Autodesk Inventor part; units mm, degrees
ref_plane "YZ Plane" through (0, 0, 0) normal (1, 0, 0) x (0, 1, 0)
ref_plane "XZ Plane" through (0, 0, 0) normal (0, 1, 0) x (-1, 0, 0)
ref_plane "XY Plane" through (0, 0, 0) normal (0, 0, 1) x (1, 0, 0)
sketch "Sketch1" plane through (0, 0, 0) normal (0, 1, 0) x (-1, 0, 0)
  line L0 (0, 0) -> (45, 0)
  line L1 (45, 0) -> (45, -20)
  line L2 (45, -20) -> (0, -20)
  line L3 (0, -20) -> (0, 0)
  circle A0 centre (39.9418, -5.8805) radius 1.5
  circle A1 centre (39.4697, -15.8219) radius 1.5
  circle A2 centre (3.2694, -6.6358) radius 1.5
  circle A3 centre (3.2694, -15.8219) radius 1.5
  dimension "d0" = 45
  dimension "d1" = 20
  dimension "d4" = 3
  dimension "d5" = 3
  dimension "d6" = 3
  dimension "d7" = 3
extrude "Extrusion1" add sketch "Sketch1" along normal blind 3 contours L0 L1 L2 L3 | A0 | A1 | A2 | A3
extrude "Extrusion2" cut sketch "Sketch1" along normal through all contours A0 | A1 | A2 | A3
sketch "Sketch2" plane through (-45, 0, 0) normal (0, 0, 1) x (1, 0, 0)
  line L0 (0, 0) -> (45, 0)
  line L1 (45, 0) -> (45, 105)
  line L2 (45, 105) -> (0, 105)
  line L3 (0, 105) -> (0, 0)
  line L4 (10.782, 97.156) -> (34.218, 97.156)
  line L5 (34.218, 97.156) -> (34.218, 84.256)
  line L6 (34.218, 84.256) -> (10.782, 84.256)
  line L7 (10.782, 84.256) -> (10.782, 97.156)
  circle A0 centre (8.582, 90.706) radius 1.5
  circle A1 centre (36.418, 90.706) radius 1.5
  line L8 (10.782, 79.3472) -> (34.218, 79.3472)
  line L9 (34.218, 79.3472) -> (34.218, 66.4472)
  line L10 (34.218, 66.4472) -> (10.782, 66.4472)
  line L11 (10.782, 66.4472) -> (10.782, 79.3472)
  circle A2 centre (8.582, 72.8972) radius 1.5
  circle A3 centre (36.418, 72.8972) radius 1.5
  line L12 (10.782, 61.5315) -> (34.218, 61.5315)
  line L13 (34.218, 61.5315) -> (34.218, 48.6315)
  line L14 (34.218, 48.6315) -> (10.782, 48.6315)
  line L15 (10.782, 48.6315) -> (10.782, 61.5315)
  circle A4 centre (8.582, 55.0815) radius 1.5
  circle A5 centre (36.418, 55.0815) radius 1.5
  circle A6 centre (36.418, 37.2658) radius 1.5
  circle A7 centre (8.582, 37.2658) radius 1.5
  line L16 (10.782, 30.8158) -> (10.782, 43.7158)
  line L17 (34.218, 30.8158) -> (10.782, 30.8158)
  line L18 (34.218, 43.7158) -> (34.218, 30.8158)
  line L19 (10.782, 43.7158) -> (34.218, 43.7158)
  line L20 (10.782, 97.156) -> (34.218, 97.156)
  line L21 (34.218, 97.156) -> (34.218, 24.1177)
  line L22 (34.218, 24.1177) -> (10.782, 24.1177)
  line L23 (10.782, 24.1177) -> (10.782, 97.156)
  circle A8 centre (8.582, 85.7719) radius 1.5
  circle A9 centre (36.418, 85.7719) radius 1.5
  circle A10 centre (8.582, 79.3472) radius 1.5
  circle A11 centre (36.418, 79.3472) radius 1.5
  circle A12 centre (8.582, 66.4472) radius 1.5
  circle A13 centre (36.418, 66.4472) radius 1.5
  circle A14 centre (36.418, 46.9762) radius 1.5
  circle A15 centre (8.582, 46.9762) radius 1.5
  point P0 (10.782, 90.706)
  point P1 (10.782, 72.8972)
  point P2 (10.782, 55.0815)
  point P3 (10.782, 37.2658)
  dimension "d10" = 105
  dimension "d13" = 45
  dimension "d14" = 23.436
  dimension "d15" = 12.9
  dimension "d17" = 10.782
  dimension "d18" = 3
  dimension "d19" = 3
  dimension "d20" = 2.2
  dimension "d21" = 2.2
  dimension "d22" = 23.436
  dimension "d23" = 12.9
  dimension "d24" = 3
  dimension "d25" = 3
  dimension "d26" = 2.2
  dimension "d27" = 2.2
  dimension "d28" = 23.436
  dimension "d29" = 12.9
  dimension "d30" = 3
  dimension "d31" = 3
  dimension "d32" = 2.2
  dimension "d33" = 2.2
  dimension "d34" = 23.436
  dimension "d35" = 12.9
  dimension "d36" = 3
  dimension "d37" = 3
  dimension "d38" = 2.2
  dimension "d39" = 2.2
  dimension "d44" = 3
  dimension "d45" = 3
  dimension "d46" = 3
  dimension "d47" = 3
  dimension "d48" = 3
  dimension "d49" = 3
  dimension "d50" = 3
  dimension "d51" = 3
extrude "Extrusion3" add sketch "Sketch2" along normal blind 3 contours L3 L2 L1 L0 | L4 L5 L6 L7 | L6 L21 L8 L23 | L8 L9 L10 L11 | L10 L21 L12 L23 | L12 L13 L14 L15 | L14 L21 L19 L23 | L19 L18 L17 L16 | L17 L21 L22 L23 | A0 | A1 | A2 | A3 | A4 | A5 | A6 | A7 | A8 | A9 | A10 | A11 | A12 | A13 | A14 | A15
extrude "Extrusion4" cut sketch "Sketch2" along normal through all contours L4 L5 L6 L7 | L8 L9 L10 L11 | L12 L13 L14 L15 | L19 L18 L17 L16 | A0 | A1 | A2 | A3 | A4 | A5 | A6 | A7
extrude "Extrusion5" cut sketch "Sketch2" along normal through all contours L6 L21 L8 L23 | L10 L21 L12 L23 | L14 L21 L19 L23 | L17 L21 L22 L23
extrude "Extrusion6" cut sketch "Sketch2" along normal blind 3 contours A8 | A9 | A10 | A11 | A12 | A13 | A14 | A15
fillet "Fillet1" radius 5 1 edges at (-45, 105, 1.5)
fillet "Fillet2" radius 5 1 edges at (0, 105, 1.5)
fillet "Fillet3" radius 2 2 edges at (0, 1.5, -20) (-45, 1.5, -20)
sketch "Sketch4" plane through (-45, 0, 3) normal (0, 0, 1) x (1, 0, 0)
  point P0 (45, 0)
equation "\"d52\" = d48"
properties part number "servo atach"
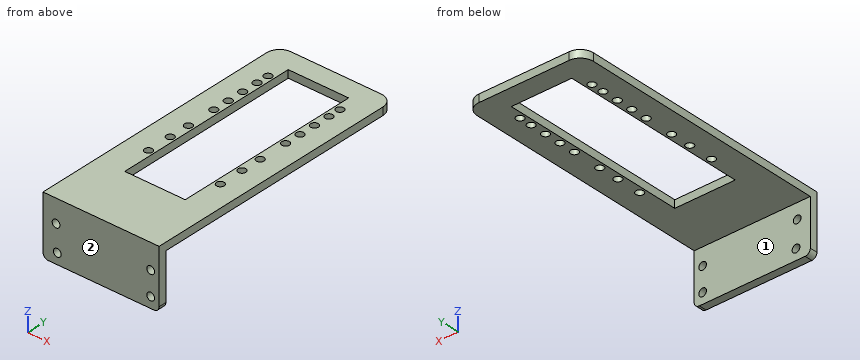
Geometry check sheet. Reference: the model listing, model coordinates, mm. Face numbers are marked on the shaded views. A direction names the side the tool comes from. Coordinates: 2 decimals unless noted, no trailing zeros. Order: outer loops, then holes, each group sorted by start corner. A loop starts at its lowest first (then second) coordinate and runs counter-clockwise, first axis right, second up. Notation, with made-up numbers: (0, -4) - (41, -4) arc R20 cw to (41, 32) - close; hole circle Ø6 at (-22, 22.25). An arc over 180 degrees is marked (long way). Answer in a Markdown table with one row per item. Add a question column.
1. Material ranges on L1, parallel to X at y = 41.5, z = 2; L2, parallel to Y at x = -17.5, z = -18.25, recorded low to high. Write a range as [from, to].
2. Access from +Z, -Z, +X, -X, +Y, -Y to the whole of each face (thin tool, end or side, straight path). Record for the marked faces 1 and 2.
3. Gauge pin test, flat ends, axial feed: pin 1 Ø13.5 at (x, y) = (-15.5, 35.5) entering from -Z; pin 2 Ø4 at (x, z) = (-9.5, -5.5) entering from +Y. Record the tip position at first contact, or that the pin passes through.
4. Section check B-B (x = -23.5). Enter the section's corners in (y, z), plus the area to 3 significant figures.
5. Section check C-C (z = -9.75). Enter the section's corners in (x, y), plus the area to 3 significant figures.
6. Section check A-A (y = 83). Enter the section's corners in (x, z).
Data:
| question | item | result |
|---|---|---|
| 1 | L1 | x = [-45, -34.22], [-10.78, 0] |
| 1 | L2 | y = [0, 3] |
| 2 | face 1 | -Z, +X, -X, +Y |
| 2 | face 2 | +Z, -Z, +X, -X, -Y |
| 3 | pin 1 | stops at z = 0 |
| 3 | pin 2 | stops at y = 3 |
| 4 | outline | (0, -20) - (3, -20) - (3, 0) - (24.12, 0) - (24.12, 3) - (0, 3) - close; (97.16, 0) - (105, 0) - (105, 3) - (97.16, 3) - close |
| 4 | area | 156 mm² |
| 5 | outline | (-45, 0) - (0, 0) - (0, 3) - (-45, 3) - close |
| 5 | area | 135 mm² |
| 6 | outline | (-45, 0) - (-34.22, 0) - (-34.22, 3) - (-45, 3) - close; (-10.78, 0) - (0, 0) - (0, 3) - (-10.78, 3) - close |
